Part model, mm, in its own coordinate system. Give positions to 0.01 mm unless a question says otherwise; leave off trailing zeros. Write each loop counter-clockwise with the first axis right and the second up, starting at its lowest first coordinate (ties: lowest second). Pieces come first, ordered by that corner, then holes.
from build123d import *

# Parameters (mm, degrees)
SKETCH_1_W      = 46
SKETCH_1_H      = 25.8
EXTRUDE_1_DEPTH = 8
FILLET_1_R      = 3.2


with BuildPart() as part:
    # 草图1 → 凸台-拉伸1 (new body)
    with BuildSketch(Plane(origin=(0, 0, 0), x_dir=(1, 0, 0), z_dir=(0, 1, 0))):
        Rectangle(SKETCH_1_W, SKETCH_1_H)
    extrude(amount=EXTRUDE_1_DEPTH)

    # 圆角1
    fillet_1_edges = [part.edges().sort_by_distance(p)[0] for p in [
        (0, 8, -12.9),
        (-23, 8, 0),
        (0, 0, -12.9),
        (0, 0, 12.9),
        (-23, 0, 0),
        (0, 8, 12.9),
    ]]
    fillet(fillet_1_edges, radius=FILLET_1_R)


solid = part.part
1) Saw through at A-A (x = -16.5). Write the cut outline in (y, z).
Check result:
outline: (0, -9.7) arc R3.2 ccw to (3.2, -12.9) - (4.8, -12.9) arc R3.2 ccw to (8, -9.7) - (8, 9.7) arc R3.2 ccw to (4.8, 12.9) - (3.2, 12.9) arc R3.2 ccw to (0, 9.7) - close
2) Drill centre lines: L1, parallel to Z at x = 19, y = 3; L2, parallel to X at y = 1, z = -10; L3, parallel to Z at x = 7.5, y = 1.75. Where is each one in solid material? Low to high.
Check result:
L1: z = -12.89 to 12.89
L2: x = -22.12 to 23
L3: z = -12.55 to 12.55
3) Saw through at B-B (y = 2). Write the cut outline in (x, z).
Check result:
outline: (-22.77, -12.67) - (23, -12.67) - (23, 12.67) - (-22.77, 12.67) - close
4) Saw through at C-C (z = -11). Write the cut outline in (x, y).
Check result:
outline: (-23, 3.2) arc R3.2 ccw to (-21.1, 0.28) - (23, 0.28) - (23, 7.72) - (-21.1, 7.72) arc R3.2 ccw to (-23, 4.8) - close
5) Saw through at D-D (y = 6.75). Write the cut outline in (x, z).
Check result:
outline: (-22.34, -12.24) - (23, -12.24) - (23, 12.24) - (-22.34, 12.24) - close
6) Flat gauge pin, fed straight in: P1, Ø2, axis at y = 1.5, z = -3, coming from the -X side. Where does the tip first touch, or does it go through?
Check result:
P1: stops at x = -22.92
